```python
from build123d import *

# Parameters (mm, degrees)
F0_R     = 1.7
F0_R_2   = 2.65
F1_DEPTH = 1.7
F2_R     = 2.65
F3_DEPTH = 2
F4_R     = 3.15
F5_DEPTH = 6
F6_SIZE  = 1
F7_R     = 2.4
F8_DEPTH = 5


with BuildPart() as f1:
    # F0 (on Top) → F1 (new body)
    with BuildSketch(Plane.XY):
        with BuildLine():
            Line((1.393512, -2.825), (8, -2.825))
            Line((8, -2.825), (8, 2.825))
            Line((8, 2.825), (1.393512, 2.825))
            ThreePointArc((1.393512, 2.825), (2.675076, 1.663271), (3.15, 0))
            ThreePointArc((3.15, 0), (2.675076, -1.663271), (1.393512, -2.825))
        make_face()
        with Locations((6, 0)):
            Circle(F0_R, mode=Mode.SUBTRACT)
        with BuildLine():
            Line((-8, -2.825), (-1.393512, -2.825))
            ThreePointArc((-1.393512, -2.825), (-3.15, 0), (-1.393512, 2.825))
            Line((-1.393512, 2.825), (-8, 2.825))
            Line((-8, 2.825), (-8, -2.825))
        make_face()
        with Locations((-6, 0)):
            Circle(F0_R, mode=Mode.SUBTRACT)
        with BuildLine():
            Line((-1.393512, -2.825), (1.393512, -2.825))
            ThreePointArc((1.393512, -2.825), (2.675076, -1.663271), (3.15, 0))
            ThreePointArc((3.15, 0), (2.675076, 1.663271), (1.393512, 2.825))
            Line((1.393512, 2.825), (-1.393512, 2.825))
            ThreePointArc((-1.393512, 2.825), (-3.15, 0), (-1.393512, -2.825))
        make_face()
        Circle(F0_R_2, mode=Mode.SUBTRACT)
        Circle(F0_R_2)
    extrude(amount=F1_DEPTH)

    # F2 (on face) → F3 (join)
    with BuildSketch(Plane.XY.offset(1.7)):
        Circle(F2_R)
    extrude(amount=F3_DEPTH)

    # F4 (on face) → F5 (join)
    with BuildSketch(Plane.XY.offset(3.7)):
        Circle(F4_R)
    extrude(amount=F5_DEPTH)

    # F6
    f6_edges = [f1.edges().sort_by_distance(p)[0] for p in [
        (-8, -2.825, 0.85),
        (-8, 2.825, 0.85),
        (8, -2.825, 0.85),
        (8, 2.825, 0.85),
    ]]
    chamfer(f6_edges, length=F6_SIZE)

    # F7 (on face) → F8 (join)
    with BuildSketch(Plane.XY):
        Circle(F7_R)
    extrude(amount=-F8_DEPTH)


solid = f1.part
```
Model file for the job. Use its own axes, mm. A direction names the side the tool comes from. Coordinates: 2 decimals unless noted, no trailing zeros. Order: outer loops, then holes, each group sorted by start corner. A loop starts at its lowest first (then second) coordinate and runs counter-clockwise, first axis right, second up. Notation, with made-up numbers: (14.5, 29.25) -> (67.5, 29.25) arc R24 ccw to (67.5, 64.25) -> close; hole circle Ø9 at (-16, -3). An arc over 180 degrees is marked (long way). Answer as a JSON object with one key per item and string values. Group by question number.
1) Which spindle directions (+Z, -Z, +X, -X, +Y, -Y) get a long thin tool onto all of the face, cutting with end or side? Do faces 1 (the face through (-2.5, -1.917, 6.658)), 2 (the face through (-2, 2, 3.7)), 3 (the face through (1.29, 2.024, -2.465)). Say none if no direction does.
2) Cut at B-B, the plane x = 6. Write the cut outline in (y, z) (3 decimals), then the cut area to 4 significant figures.
3) Drill centre lines: L1, parallel to Y at x = 6, z = 0.5 (3 decimals); L2, parallel to Z at x = -4.5, y = -1.75; L3, parallel to Y at x = -4.25, z = 1.25 (3 decimals). Where is each one in solid material? Low to high.
4) Cut at D-D, the plane z = 5. Write the cut outline in (x, y).
5) Pull direction Y, two halves, no side cores. Call faces 4 (the face through (2.45, -1.01, 2.69)), 5 (the face through (4.65, -1.03, 0.84)), 6 (the face through (-7.507, -2.318, 0.838)): +Y half, -Y half, draft (parallel to the pull), parting line (faces both ways), or undercut.
6) Flat gauge pins, fed straight in: pin 1 (2 mm diameter, centred on x = -5.5, z = 7, fed in from +Y); pin 2 (2 mm diameter, centred on x = 4.5, z = 0.5, fed in from -Y) (3 decimals); pin 3 (1.4 mm diameter, centred on x = 2.5, z = 0.5, fed in from +Y) (3 decimals). Where does each tip first touch, or does it go through?
7) Cut at A-A, the plane y = 0. Write the cut outline in (x, z).
8) Cut at C-C, the plane x = -0.5. Write the cut outline in (y, z) (3 decimals), then the cut area to 3 significant figures.
Check values:
{
 "1": {"face 1": "+Z", "face 2": "none", "face 3": "-Z"},
 "2": {"outline": "(-2.825, 0) -> (-1.7, 0) -> (-1.7, 1.7) -> (-2.825, 1.7) -> close; (1.7, 0) -> (2.825, 0) -> (2.825, 1.7) -> (1.7, 1.7) -> close", "area": "3.825 mm²"},
 "3": {"L1": "y = -2.825 to -1.7, 1.7 to 2.825", "L2": "z = 0 to 1.7", "L3": "y = -2.825 to 2.825"},
 "4": {"outline": "circle Ø6.3 at (0, 0)"},
 "5": {"face 4": "parting line", "face 5": "undercut", "face 6": "-Y half"},
 "6": {"pin 1": "passes through", "pin 2": "stops at y = -2.825", "pin 3": "stops at y = 2.825"},
 "7": {"outline": "(-8, 0) -> (-7.7, 0) -> (-7.7, 1.7) -> (-8, 1.7) -> close; (-4.3, 0) -> (-2.4, 0) -> (-2.4, -5) -> (2.4, -5) -> (2.4, 0) -> (4.3, 0) -> (4.3, 1.7) -> (2.65, 1.7) -> (2.65, 3.7) -> (3.15, 3.7) -> (3.15, 9.7) -> (-3.15, 9.7) -> (-3.15, 3.7) -> (-2.65, 3.7) -> (-2.65, 1.7) -> (-4.3, 1.7) -> close; (7.7, 0) -> (8, 0) -> (8, 1.7) -> (7.7, 1.7) -> close"},
 "8": {"outline": "(-3.11, 3.7) -> (-2.602, 3.7) -> (-2.602, 1.7) -> (-2.825, 1.7) -> (-2.825, 0) -> (-2.347, 0) -> (-2.347, -5) -> (2.347, -5) -> (2.347, 0) -> (2.825, 0) -> (2.825, 1.7) -> (2.602, 1.7) -> (2.602, 3.7) -> (3.11, 3.7) -> (3.11, 9.7) -> (-3.11, 9.7) -> close", "area": "80.8 mm²"}
}
